from build123d import *

# Parameters (mm, degrees)
F0_R     = 158.75
F0_R_2   = 11.1125
F0_R_3   = 84.1375
F1_DEPTH = 35.052
F2_R     = 101.6
F2_R_2   = 84.1375
F3_DEPTH = 1.905
F4_R     = 1.90499


# Not quite as in the source:
# - a fillet or chamfer is up to 0.001 mm smaller than in the source, because OpenCascade refuses the exact size


with BuildPart() as f1:
    # F0 (on Front) → F1 (new body)
    with BuildSketch(Plane.XZ):
        Circle(F0_R)
        with Locations((-51.6140452568, -124.6073280679)):
            Circle(F0_R_2, mode=Mode.SUBTRACT)
        with Locations((-124.6073280679, -51.6140452568)):
            Circle(F0_R_2, mode=Mode.SUBTRACT)
        with Locations((51.6140452568, -124.6073280679)):
            Circle(F0_R_2, mode=Mode.SUBTRACT)
        with Locations((124.6073280679, -51.6140452568)):
            Circle(F0_R_2, mode=Mode.SUBTRACT)
        with Locations((-124.6073280679, 51.6140452568)):
            Circle(F0_R_2, mode=Mode.SUBTRACT)
        with Locations((-51.6140452568, 124.6073280679)):
            Circle(F0_R_2, mode=Mode.SUBTRACT)
        Circle(F0_R_3, mode=Mode.SUBTRACT)
        with Locations((124.6073280679, 51.6140452568)):
            Circle(F0_R_2, mode=Mode.SUBTRACT)
        with Locations((51.6140452568, 124.6073280679)):
            Circle(F0_R_2, mode=Mode.SUBTRACT)
    extrude(amount=F1_DEPTH)

    # F2 (on face) → F3 (join)
    with BuildSketch(Plane.XZ.offset(35.052)):
        Circle(F2_R)
        Circle(F2_R_2, mode=Mode.SUBTRACT)
    extrude(amount=F3_DEPTH)

    # F4 (radius 1.905 in the source; OpenCascade refuses exactly that, so slightly less here)
    f4_edges = [f1.edges().sort_by_distance(p)[0] for p in [
        (-158.75, -35.052, 0),
        (-158.75, 0, 0),
        (-101.6, -36.957, 0),
    ]]
    fillet(f4_edges, radius=F4_R)


solid = f1.part
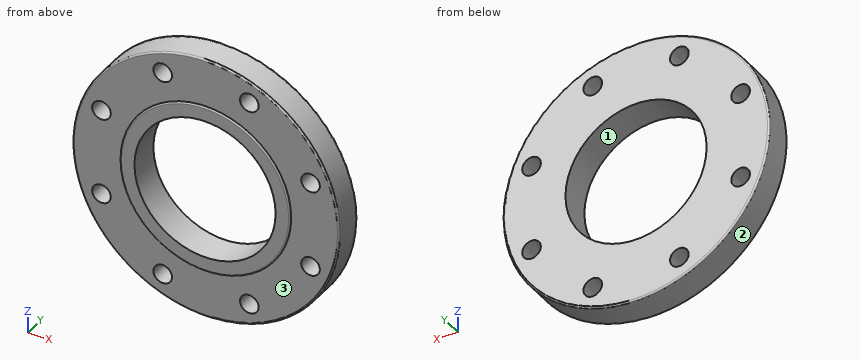
Source: CAD feature listing. Evaluate the final solid. Frame: model axes, mm. Face numbers are marked on the shaded views. Give positions to 0.01 mm unless a question says otherwise; leave off trailing zeros. Use a Markdown table: item, result.
1) Mould query, pull axis X, two halves, no side actions, for the marked faces 1, 2 and 3. Classes: +X half, -X half, draft (parallel to the pull), parting line (faces both ways), or undercut.
Answer list:
| item | result |
|---|---|
| face 1 | undercut |
| face 2 | parting line |
| face 3 | draft |
2) Contact query for flat-ended pins moving along their axis: P1, Ø4, axis at x = -43, y = -16, coming from the +Z side; P2, Ø4, axis at x = 32.5, y = -8.5, coming from the +Z side; P3, Ø12, axis at x = -31, y = -24, coming from the +Z side. Output: stop coordinate, or through.
Answer list:
| item | result |
|---|---|
| P1 | z = 153.36 |
| P2 | z = 155.79 |
| P3 | z = 156.77 |
3) Section query C-C, the plane y = -11.5. Count the separate pieces of the cut face and the enclosed holes in it, then the cut area to 3 significant figures.
Answer list:
| item | result |
|---|---|
| separate pieces | 1 |
| enclosed holes | 9 |
| area | 53,800 mm² |
4) Ray query, line 1 along Z through (x, y) = (-53, -11.5); line 2 along Z through (x, y) = (48, -21.5). Return the intervals inside material, ascending. Write a range as [from, to].
Answer list:
| item | result |
|---|---|
| line 1 | [-149.64, -135.63], [-113.58, -65.35], [65.35, 113.58], [135.63, 149.64] |
| line 2 | [-151.32, -135.12], [-114.1, -69.1], [69.1, 114.1], [135.12, 151.32] |
